The model under review builds one solid part; all positions refer to its coordinate system, in mm. Face numbers are marked on the shaded views. A direction names the side the tool comes from. Round coordinates to 2 decimals unless told otherwise and drop trailing zeros. Order: outer loops, then holes, each group sorted by start corner. A loop starts at its lowest first (then second) coordinate and runs counter-clockwise, first axis right, second up. Notation, with made-up numbers: M 9.25,41.25 L 47.25,41.25 A19 ccw 47.25,71.25 Z; hole C -15,2 d2. An arc over 180 degrees is marked long. Answer as a JSON object with one key per item and string values. Group by question number.
1. Add section C-C on z = 1.75. State the section outline as (x, y) points.
2. Machinability: for the marked faces 1, 2 and 3, which of the approach directions +Z, -Z, +X, -X, +Y, -Y give a long, thin tool a straight path to every point of the face, cutting with its end or side? Answer none if there is none.
3. To check wall thickness, follow probe 1 along Y at (x, z) = (-0.75, 2.6); probe 2 along Z at (x, y) = (3.5, -1.15); probe 3 along Z at (x, y) = (-4.5, 1.6). State the ranges of each line that lie inside material, in increasing order. Write a range as [from, to].
4. Add section B-B on z = -0.45. State the section outline as (x, y) points (3 decimals).
5. Add section A-A on x = 1. State the section outline as (y, z) points, and give its area (3 significant figures).
6. Add section D-D on x = 2.4. State the section outline as (y, z) points (3 decimals), and give its area (3 significant figures).
7. Clearance check with flat-ended pins moving along their axes: P1, Ø3, axis at x = 0, z = -1, coming from the +Y side; P2, Ø0.8, axis at x = 0, z = 1, coming from the +Y side; P3, Ø0.8, axis at x = -0.5, z = 2.5, coming from the -Y side; P4, Ø2, axis at y = 1, z = 2, coming from the -X side. State where each tip first meets the part, or that it passes through.
```python
from build123d import *

# Parameters (mm, degrees)
F1_DEPTH  = 0.2
F3_DEPTH  = 0.2
F5_DEPTH  = 3.1
F8_R      = 0.5
F9_R      = 0.215
F10_DEPTH = 2


with BuildPart() as f1:
    # F0 (on Top) → F1 (new body)
    with BuildSketch(Plane.XY):
        with BuildLine():
            Line((0, 2.15), (0, 0))
            Line((0, 0), (5.35, 0))
            ThreePointArc((5.35, 0), (4.72028, 1.52028), (3.2, 2.15))
            Line((3.2, 2.15), (0, 2.15))
        make_face()
    extrude(amount=F1_DEPTH)

    # F2 (on face) → F3 (join)
    with BuildSketch(Plane.XY.offset(0.2)):
        with BuildLine():
            Line((0, 0), (5.15, 0))
            ThreePointArc((5.15, 0), (4.578858, 1.378858), (3.2, 1.95))
            Line((3.2, 1.95), (0, 1.95))
            Line((0, 1.95), (0, 0))
        make_face()
    extrude(amount=F3_DEPTH)

    # F4 (on face) → F5 (join)
    with BuildSketch(Plane.XY.offset(0.4)):
        with BuildLine():
            Line((0, 0), (4.95, 0))
            ThreePointArc((4.95, 0), (4.437437, 1.237437), (3.2, 1.75))
            Line((3.2, 1.75), (0, 1.75))
            Line((0, 1.75), (0, 0))
        make_face()
    extrude(amount=F5_DEPTH)

    # F6: F1 across face


with BuildPart() as f1_1:
    add(f1.part)
    add(f1.part.mirror(Plane(origin=(0, 0.895016, 1.719576), x_dir=(0, -1, 0), z_dir=(-1, 0, 0))))

    # F7: F1 across face


with BuildPart() as f1_2:
    add(f1_1.part)
    add(f1_1.part.mirror(Plane(origin=(0, 0, 1.739109), x_dir=(1, 0, 0), z_dir=(0, -1, 0))))

    # F8
    f8_edges = [f1_2.edges().sort_by_distance(p)[0] for p in [
        (0, 1.75, 3.5),
        (-4.95, 0, 3.5),
        (0, -1.75, 3.5),
        (4.95, 0, 3.5),
    ]]
    fillet(f8_edges, radius=F8_R)

    # F9 (on face) → F10 (join)
    with BuildSketch(Plane(origin=(0, 0, 0), x_dir=(1, 0, 0), z_dir=(0, 0, -1))):
        with Locations((2.4, 0)):
            Circle(F9_R)
        with Locations((-2.4, 0)):
            Circle(F9_R)
    extrude(amount=F10_DEPTH)


solid = f1_2.part
```
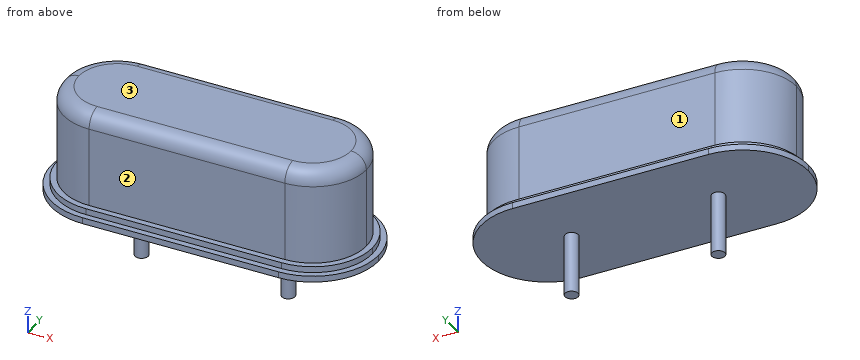
Recorded:
{
 "1": {"outline": "M -3.2,-1.75 L 3.2,-1.75 A1.75 ccw 3.2,1.75 L -3.2,1.75 A1.75 ccw Z"},
 "2": {"face 1": "+Z, +X, -X, +Y", "face 2": "+Z, +X, -X, -Y", "face 3": "+Z, +X, -X, +Y, -Y"},
 "3": {"probe 1": "y = [-1.75, 1.75]", "probe 2": "z = [0, 3.5]", "probe 3": "z = [0, 0.2]"},
 "4": {"outline": "C -2.4,0 d0.43; C 2.4,0 d0.43"},
 "5": {"outline": "M -2.15,0 L 2.15,0 L 2.15,0.2 L 1.95,0.2 L 1.95,0.4 L 1.75,0.4 L 1.75,3 A0.5 ccw 1.25,3.5 L -1.25,3.5 A0.5 ccw -1.75,3 L -1.75,0.4 L -1.95,0.4 L -1.95,0.2 L -2.15,0.2 Z", "area": "12.4 mm²"},
 "6": {"outline": "M -2.15,0 L -0.215,0 L -0.215,-2 L 0.215,-2 L 0.215,0 L 2.15,0 L 2.15,0.2 L 1.95,0.2 L 1.95,0.4 L 1.75,0.4 L 1.75,3 A0.5 ccw 1.25,3.5 L -1.25,3.5 A0.5 ccw -1.75,3 L -1.75,0.4 L -1.95,0.4 L -1.95,0.2 L -2.15,0.2 Z", "area": "13.2 mm²"},
 "7": {"P1": "stops at y = 2.15", "P2": "stops at y = 1.75", "P3": "stops at y = -1.75", "P4": "stops at x = -4.95"}
}
